Geometry check sheet. Reference: the model listing, model coordinates, mm. Face numbers are marked on the shaded views. A direction names the side the tool comes from. Round coordinates to 2 decimals unless told otherwise and drop trailing zeros. Loops run counter-clockwise (first coordinate to the right, second up) from the corner with the lowest first, then second, coordinate; pieces in that order, holes last. Notation, with made-up numbers: (-36, 85.25) - (-11, 85.25) arc R29 cw to (-11, 113.25) - close; hole circle Ø3 at (-18.75, 4). An arc over 180 degrees is marked (long way). Answer as CSV lines item,"result". Start each with the question number.
1) Depth check by flat-ended pin: P1, Ø2.5, axis at x = 16, y = -16, coming from the -Z side; P2, Ø6, axis at x = -7, z = -4.5, coming from the -Y side. Enter the tip coordinate at first touch or a pass-through.
2) Cross-section at D-D on z = -8. Record the boundary of the cut face in (x, y).
3) Cross-section at B-B on z = -13. Record the boundary of the cut face in (x, y).
4) Thickness scan on line 1 along X through (y, z) = (-13.5, 1.25); line 2 along X through (y, z) = (5.4, -13); line 3 along Y through (x, z) = (17, -0.5). Record the ranges inside material, lowest first.
5) Access from +Z, -Z, +X, -X, +Y, -Y to the whole of each face (thin tool, end or side, straight path). Record for the marked faces 1 and 2.
6) Cross-section at A-A on y = -24. Record the boundary of the cut face in (x, z).
7) Cross-section at C-C on x = 18.5. Record the boundary of the cut face in (y, z), and give its area (3 significant figures).
from build123d import *

# Parameters (mm, degrees)
SKETCH3_W             = 9
SKETCH3_H             = 40
SKETCH3_R             = 1.5
BOSS_EXTRUDE5_DEPTH   = 2
BOSS_EXTRUDE5_2_DEPTH = 2
SKETCH5_W             = 46
SKETCH5_H             = 20
SKETCH5_R             = 1.5
BOSS_EXTRUDE7_DEPTH   = 2


with BuildPart() as part:
    # Sketch3 → Boss-Extrude5 (new body)
    with BuildSketch(Plane.XY):
        with Locations((-21.015808288, -14.438328765)):
            Rectangle(SKETCH3_W, SKETCH3_H)
        with Locations((-21.015808288, -29.438328765)):
            Circle(SKETCH3_R, mode=Mode.SUBTRACT)
        with Locations((-21.015808288, -6.938328765)):
            Circle(SKETCH3_R, mode=Mode.SUBTRACT)
    extrude(amount=BOSS_EXTRUDE5_DEPTH)



with BuildPart() as body_2:
    # Sketch3 → Boss-Extrude5 2 (new body)
    with BuildSketch(Plane.XY):
        with Locations((15.984191712, -14.438328765)):
            Rectangle(SKETCH3_W, SKETCH3_H)
        with Locations((15.984191712, -29.438328765)):
            Circle(SKETCH3_R, mode=Mode.SUBTRACT)
        with Locations((15.984191712, -6.938328765)):
            Circle(SKETCH3_R, mode=Mode.SUBTRACT)
    extrude(amount=BOSS_EXTRUDE5_2_DEPTH)


with BuildPart() as part_1:
    add(part.part)

    add(body_2.part)  # Boss-Extrude7 merges body 2
    # Sketch5 → Boss-Extrude7 (add)
    with BuildSketch(Plane(origin=(0, 4, 0), x_dir=(1, 0, 0), z_dir=(0, 1, 0))):
        with Locations((-2.515808288, 8)):
            Rectangle(SKETCH5_W, SKETCH5_H)
        with Locations(Location((-2.515808288, 13, 0), (0, 0, 270))):
            Circle(SKETCH5_R, mode=Mode.SUBTRACT)
    extrude(amount=BOSS_EXTRUDE7_DEPTH)


solid = part_1.part
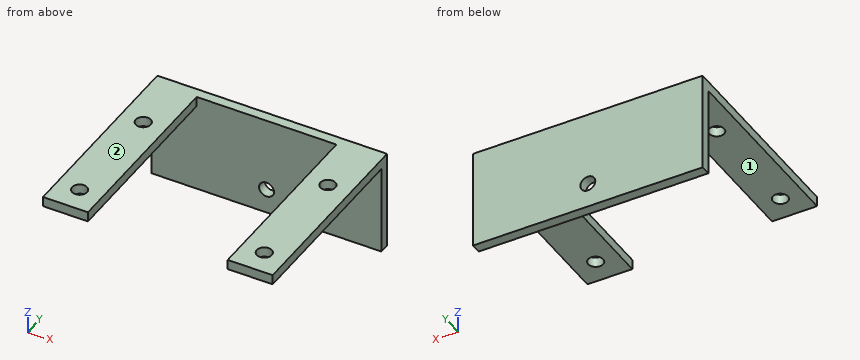
Answer block:
1,P1,"stops at z = 0"
1,P2,"stops at y = 4"
2,outline,"(-25.52, 4) - (20.48, 4) - (20.48, 6) - (-25.52, 6) - close"
3,outline,"(-25.52, 4) - (-4.02, 4) - (-4.02, 6) - (-25.52, 6) - close; (-1.02, 4) - (20.48, 4) - (20.48, 6) - (-1.02, 6) - close"
4,line 1,"x = -25.52 to -16.52, 11.48 to 20.48"
4,line 2,"x = -25.52 to -4.02, -1.02 to 20.48"
4,line 3,"y = 4 to 6"
5,face 1,"-Z, +X, -X, -Y"
5,face 2,"+Z, +X, -X, +Y, -Y"
6,outline,"(-25.52, 0) - (-16.52, 0) - (-16.52, 2) - (-25.52, 2) - close; (11.48, 0) - (20.48, 0) - (20.48, 2) - (11.48, 2) - close"
7,outline,"(-34.44, 0) - (4, 0) - (4, -18) - (6, -18) - (6, 2) - (-34.44, 2) - close"
7,area,"117 mm^2"
